from build123d import *

# Parameters (mm, degrees)
F0_R     = 4.445
F1_DEPTH = 9.525
F2_R     = 6.35
F2_R_2   = 4.445
F3_DEPTH = 1.27
F4_R     = 0.3175


with BuildPart() as f1:
    # F0 (on Top) → F1 (new body)
    with BuildSketch(Plane.XY):
        Circle(F0_R)
    extrude(amount=F1_DEPTH)

    # F2 (on face) → F3 (join)
    with BuildSketch(Plane.XY.offset(9.525)):
        Circle(F2_R)
        Circle(F2_R_2, mode=Mode.SUBTRACT)
    extrude(amount=-F3_DEPTH)

    # F4
    f4_edges = [f1.edges().sort_by_distance(p)[0] for p in [
        (-6.35, 0, 9.525),
    ]]
    fillet(f4_edges, radius=F4_R)


solid = f1.part
Verification items for the finished model (mm, model axes). A direction names the side the tool comes from. Give positions to 0.01 mm unless a question says otherwise; leave off trailing zeros. Order: outer loops, then holes, each group sorted by start corner. A loop starts at its lowest first (then second) coordinate and runs counter-clockwise, first axis right, second up. Notation, with made-up numbers: M 23,83 L 27,83 A18 cw 27,91 Z; hole C -17.75,-39.75 d4. An arc over 180 degrees is marked long. Answer as a JSON object with one key per item and string values. Group by question number.
1) Scan lines: line 1 along Z through (x, y) = (2.5, 5) (3 decimals); line 2 along Y through (x, z) = (-1, 6.5); line 3 along X through (y, z) = (2.25, 2.75). Record each from-to range of solid material in increasing order. Write a range as [from, to].
2) Depth check by flat-ended pin: pin 1 Ø4 at (x, z) = (-2, 2) entering from +Y (3 decimals); pin 2 Ø2 at (x, z) = (-4.5, 5.5) entering from -Y; pin 3 Ø3 at (x, z) = (3, 1) entering from +Y. Enter the tip coordinate at first touch or a pass-through.
3) Access from +Z, -Z, +X, -X, +Y, -Y to the whole of each face (thin tool, end or side, straight path). Record for faces 1 (the face through (-0.96, -4.34, 4.07)), 2 (the face through (-1.38, -6.2, 8.74)).
4) Cross-section at C-C (z = 3). Enter the section's corners in (x, y) (3 decimals), then the cut area to 3 significant figures.
Result sheet:
{
 "1": {"line 1": "z = [8.255, 9.525]", "line 2": "y = [-4.33, 4.33]", "line 3": "x = [-3.83, 3.83]"},
 "2": {"pin 1": "stops at y = 4.445", "pin 2": "stops at y = -2.74", "pin 3": "stops at y = 4.18"},
 "3": {"face 1": "-Z", "face 2": "+Z, -Z"},
 "4": {"outline": "C 0,0 d8.89", "area": "62.1 mm2"}
}
